Autodesk Inventor part; units mm, degrees
ref_plane "YZ Plane" through (0, 0, 0) normal (1, 0, 0) x (0, 1, 0)
ref_plane "XZ Plane" through (0, 0, 0) normal (0, 1, 0) x (-1, 0, 0)
ref_plane "XY Plane" through (0, 0, 0) normal (0, 0, 1) x (1, 0, 0)
sketch "스케치1" plane through (0, 0, 0) normal (0, 0, 1) x (1, 0, 0)
  line L0 (-17.5, 29.25) -> (17.5, 29.25)
  line L1 (17.5, 29.25) -> (17.5, -29.25)
  line L2 (17.5, -29.25) -> (-17.5, -29.25)
  line L3 (-17.5, -29.25) -> (-17.5, 29.25)
  line L4 (-17.5, 29.25) -> (17.5, -29.25) construction
  line L5 (17.5, 29.25) -> (-17.5, -29.25) construction
  line L6 (-13, -24.25) -> (13, -24.25)
  line L7 (13, -24.25) -> (13, 24.25)
  line L8 (13, 24.25) -> (-13, 24.25)
  line L9 (-13, 24.25) -> (-13, -24.25)
  line L10 (-13, -24.25) -> (13, 24.25) construction
  line L11 (13, -24.25) -> (-13, 24.25) construction
  line L12 (-9.5, 24.25) -> (9.5, 24.25)
  line L13 (9.5, 24.25) -> (9.5, -24.25)
  line L14 (9.5, -24.25) -> (-9.5, -24.25)
  line L15 (-9.5, -24.25) -> (-9.5, 24.25)
  line L16 (-9.5, 24.25) -> (9.5, -24.25) construction
  line L17 (9.5, 24.25) -> (-9.5, -24.25) construction
  line L18 (17.5, 25.75) -> (-17.5, 25.75)
  point P0 (0, 0)
  dimension "d0" = 58.5
  dimension "d1" = 35
  dimension "d2" = 26
  dimension "d3" = 48.5
  dimension "d4" = 3.5
  dimension "d10" = 1.5
extrude "돌출1" add sketch "스케치1" against normal blind 10 contours L18 L1 L2 L3 | L9 L8 L15 L6 | L15 L8 L13 L6 | L13 L8 L7 L6
extrude "돌출3" cut sketch "스케치1" against normal blind 6 contours L9 L8 L15 L6 | L15 L8 L13 L6 | L13 L8 L7 L6
sketch "스케치2" plane through (0, 0, -6) normal (0, 0, 1) x (1, 0, 0)
  circle A0 centre (10.5, 22.35) radius 1
  line L0 (10.5, 22.35) -> (-10.5, 22.35) construction
  line L1 (-13, 24.25) -> (13, 24.25) construction
  line L2 (0, 0) -> (0, 7.5455)
  circle A1 centre (-10.5, 22.35) radius 1
  line L3 (-13, 24.25) -> (13, 24.25)
  line L4 (0, 24.25) -> (0, -23.75) construction
  line L5 (0, 0.25) -> (5.5908, 0.25)
  circle A2 centre (10.5, -21.85) radius 1
  circle A3 centre (-10.5, -21.85) radius 1
  circle A4 centre (-10.5, 22.35) radius 1.9
  circle A5 centre (10.5, 22.35) radius 1.9
  circle A6 centre (10.5, -21.85) radius 1.9
  circle A7 centre (-10.5, -21.85) radius 1.9
  line L6 (-8.6, -21.85) -> (-8.6, -24.25)
  line L7 (13, -24.25) -> (-13, -24.25)
  line L8 (-10.5, -19.95) -> (-13, -19.95)
  line L9 (-13, -24.25) -> (-13, 24.25)
  line L10 (13, 24.25) -> (13, -24.25)
  line L11 (10.5, -19.95) -> (13, -19.95)
  line L12 (8.6, -21.85) -> (8.6, -24.25)
  line L13 (-8.6, 22.35) -> (-8.6, 24.75)
  line L14 (-10.5, 20.45) -> (-13, 20.45)
  line L15 (10.5, 20.45) -> (13, 20.45)
  line L16 (8.6, 22.35) -> (8.6, 24.75)
  point P0 (0, 22.35)
  point P1 (8.6, 24.25)
  point P2 (-8.6, 24.25)
  dimension "d13" = 2
  dimension "d14" = 21
  dimension "d15" = 1.9
  dimension "d16" = 48
  dimension "d17" = 3.8
  dimension "d18" = 3.8
extrude "돌출4" add sketch "스케치2" along normal blind 6 contours L3 A4 L14 L9 | L3 L13 A4 | A4 | L8 A7 L6 L7 L9 | L3 A5 L16 | A7 | L3 L10 L15 A5 | A5 | L12 A6 L11 L10 L7 | A6
sketch "스케치3" plane through (0, 0, 0) normal (0, 0, 1) x (1, 0, 0)
  line L0 (-8.6, 24.25) -> (8.6, 24.25)
  line L1 (-8.6, 24.25) -> (-13, 24.25)
  line L2 (-13, 24.25) -> (13, 24.25)
  line L3 (13, 24.25) -> (13, -24.25)
  line L4 (13, -24.25) -> (-13, -24.25)
  line L5 (-13, -24.25) -> (-13, 24.25)
  circle A0 centre (-10.5, -21.85) radius 1
  circle A1 centre (10.5, 22.35) radius 1
  circle A2 centre (10.5, -21.85) radius 1
  circle A3 centre (-10.5, 22.35) radius 1
  line L6 (-13, -19.95) -> (-13, 20.45)
  line L7 (-13, 20.45) -> (-10.5, 20.45)
  arc A4 (-10.5, 20.45) -> (-8.6, 22.35) centre (-10.5, 22.35) ccw
  line L8 (-8.6, 22.35) -> (-8.6, 24.25)
  line L9 (-8.6, 24.25) -> (8.6, 24.25)
  line L10 (8.6, 24.25) -> (8.6, 22.35)
  arc A5 (8.6, 22.35) -> (10.5, 20.45) centre (10.5, 22.35) ccw
  line L11 (10.5, 20.45) -> (13, 20.45)
  line L12 (13, 20.45) -> (13, -19.95)
  line L13 (13, -19.95) -> (10.5, -19.95)
  arc A6 (10.5, -19.95) -> (8.6, -21.85) centre (10.5, -21.85) ccw
  line L14 (8.6, -21.85) -> (8.6, -24.25)
  line L15 (8.6, -24.25) -> (-8.6, -24.25)
  line L16 (-8.6, -24.25) -> (-8.6, -21.85)
  arc A7 (-8.6, -21.85) -> (-10.5, -19.95) centre (-10.5, -21.85) ccw
  line L17 (-10.5, -19.95) -> (-13, -19.95)
  line L18 (17.5, -29.25) -> (17.5, 25.75)
  line L19 (17.5, 25.75) -> (-17.5, 25.75)
  line L20 (-17.5, 25.75) -> (-17.5, -29.25)
  line L21 (-17.5, -29.25) -> (17.5, -29.25)
  point P0 (0, 0)
  dimension "d21" = 26
  dimension "d22" = 48.5
extrude "돌출5" cut sketch "스케치3" against normal blind 1 contours L8 A4 L7 L5 L1 | L0 L10 A5 L11 L3 L13 A6 L14 L4 L16 A7 L17 L5 L7 A4 L8 | L2 L3 L11 A5 L10 | L17 A7 L16 L4 L5 | L3 L4 L14 A6 L13 | A0 | A1 | A2 | A3
sketch "스케치4" plane through (-13, -24.25, 0) normal (0, 1, 0) x (1, 0, 0)
  line L0 (8.75, 9.2) -> (17.25, 9.2)
  line L1 (17.25, 9.2) -> (17.25, 2.8)
  line L2 (17.25, 2.8) -> (8.75, 2.8)
  line L3 (8.75, 2.8) -> (8.75, 9.2)
  line L4 (4.4, 6) -> (21.6, 6)
  line L5 (8.75, 9.2) -> (17.25, 2.8) construction
  line L6 (17.25, 9.2) -> (8.75, 2.8) construction
  point P0 (13, 0)
  point P1 (13, 6)
  point P2 (17.25, 6)
  point P3 (8.75, 6)
  dimension "d25" = 8.5
  dimension "d26" = 6.4
extrude "돌출6" cut sketch "스케치4" against normal blind 5 contours L4 L1 L2 L3
fillet "모깎기2" radius 5 4 edges at (17.5, -29.25, -5) (-17.5, -29.25, -5) (17.5, 25.75, -5) (-17.5, 25.75, -5)
sketch "스케치5" plane through (0, 0, 0) normal (0, 0, 1) x (1, 0, 0)
  circle A0 centre (15.3, -20) radius 1
  line L0 (0, 0) -> (0, -10.3102)
  circle A1 centre (-15.3, -20) radius 1
  line L1 (0, 0) -> (6.1886, 0)
  circle A2 centre (15.3, 20) radius 1
  circle A3 centre (-15.3, 20) radius 1
  dimension "d30" = 2
  dimension "d31" = 20
  dimension "d32" = 15.3
extrude "돌출7" cut sketch "스케치5" against normal blind 5
chamfer "모따기1" distance 0.5 angle 45 4 edges at (-16.3, 20, 0) (14.3, 20, 0) (14.3, -20, 0) (-16.3, -20, 0)
properties part number "하우징"
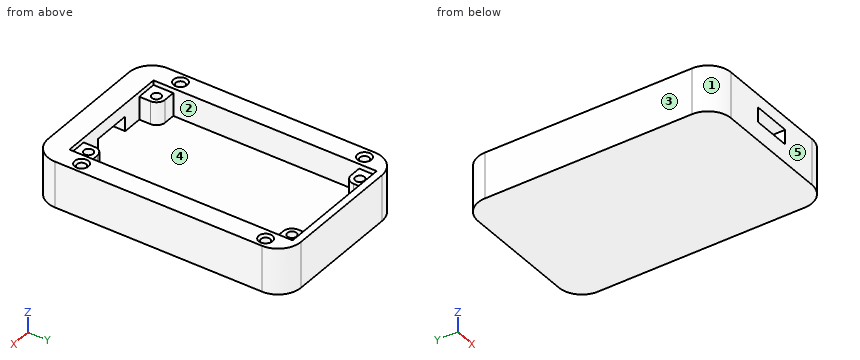
For this review, take the finished solid that the model builds, in its own axes (mm). Face numbers are marked on the shaded views. A direction names the side the tool comes from. Coordinates: 2 decimals unless noted, no trailing zeros. Loops run counter-clockwise (first coordinate to the right, second up) from the corner with the lowest first, then second, coordinate; pieces in that order, holes last. Notation, with made-up numbers: (25, -17.75) - (58, -17.75) arc R36 ccw to (58, 17.25) - close; hole circle Ø11 at (87, -18.5). An arc over 180 degrees is marked (long way). Use one line per item in the form item = value. Start each with the question number.
1) Take a section at C-C (y = 11). State the section outline as (x, z) points.
2) For pin 1 (2 mm diameter, centred on y = 23, z = -2.5, fed in from -X); pin 2 (0.6 mm diameter, centred on x = -15, y = 20.5, fed in from +Z); pin 3 (21 mm diameter, centred on x = -1.5, y = -8.5, fed in from +Z), all flat-tipped, find the tip position at first contact; note any pin that passes through.
3) Take a section at B-B (z = -1.75). State how many separate pieces and enclosed holes the cut face has, plus the area to 3 significant figures.
4) Draft analysis for pull direction Y (two halves, no side actions). For the marked faces 3, 4 and 5, state which applies: released by +Y, released by -Y, zero draft, split by the parting line, or undercut.
5) For the marked faces 1 and 2, list the 3-axis set-ups (+Z, -Z, +X, -X, +Y, -Y) from which the entire face can be reached by the end or side of a thin tool; tool diameter is ignored.
6) Take a section at D-D (x = 6). State the section outline as (y, z) points, plus the area to 3 significant figures.
7) Take a section at A-A (x = -1). State the section outline as (y, z) points.
8) To check wall thickness, follow probe 1 along X at (y, z) = (-21.85, -2.95); probe 2 along Y at (x, z) = (-10.5, -3.75); probe 3 along X at (y, z) = (16, -5.25). State the ranges of each line that lie inside material, in increasing order. Write a range as from..to.
From the geometry:
q1.outline = (-17.5, -10) - (17.5, -10) - (17.5, 0) - (13, 0) - (13, -6) - (-13, -6) - (-13, 0) - (-17.5, 0) - close
q2.pin_1 = -17.34
q2.pin_2 = -5
q2.pin_3 = -6
q3.separate_pieces = 1
q3.enclosed_holes = 9
q3.area = 686 mm2
q4.face_3 = zero draft
q4.face_4 = undercut
q4.face_5 = released by -Y
q5.face_1 = +Z, -Z, -X, -Y
q5.face_2 = +Z
q6.outline = (-29.25, -10) - (25.75, -10) - (25.75, 0) - (24.25, 0) - (24.25, -6) - (-24.25, -6) - (-24.25, 0) - (-29.25, 0) - close
q6.area = 259 mm2
q7.outline = (-29.25, -10) - (25.75, -10) - (25.75, 0) - (24.25, 0) - (24.25, -6) - (-29.25, -6) - close; (-29.25, -2.8) - (-24.25, -2.8) - (-24.25, 0) - (-29.25, 0) - close
q8.probe_1 = -17.5..-11.5, -9.5..-8.6, 8.6..9.5, 11.5..17.5
q8.probe_2 = -29.25..-22.85, -20.85..-19.95, 20.45..21.35, 23.35..25.75
q8.probe_3 = -17.5..-13, 13..17.5
